Autodesk Inventor part; units mm, degrees
ref_plane "YZ Plane" through (0, 0, 0) normal (1, 0, 0) x (0, 1, 0)
ref_plane "XZ Plane" through (0, 0, 0) normal (0, 1, 0) x (-1, 0, 0)
ref_plane "XY Plane" through (0, 0, 0) normal (0, 0, 1) x (1, 0, 0)
sketch "Sketch1" plane through (0, 0, 0) normal (0, 0, 1) x (1, 0, 0)
  line L0 (-9, 25) -> (9, 25)
  line L1 (9, 25) -> (9, -25)
  line L2 (9, -25) -> (-9, -25)
  line L3 (-9, -25) -> (-9, 25)
  point P0 (0, 0)
  point P1 (0, 25)
  point P2 (-9, 0)
  dimension "d0" = 18
  dimension "d1" = 50
extrude "Extrusion1" add sketch "Sketch1" along normal blind 3
fillet "Fillet1" radius 5 2 edges at (-9, -25, 1.5) (9, -25, 1.5)
fillet "Fillet2" radius 5 2 edges at (-9, 25, 1.5) (9, 25, 1.5)
sketch "Sketch2" plane through (0, 0, 3) normal (0, 0, 1) x (1, 0, 0)
  circle A0 centre (0, -16) radius 9
  circle A1 centre (0, 16) radius 9
  line L0 (-4, -25) -> (4, -25)
  circle A2 centre (0, -8.304) radius 0.75
  line L1 (4, 25) -> (-4, 25)
  point P0 (0, 0)
  dimension "d6" = 18
  dimension "d8" = 1.5
  dimension "d10" = 18
extrude "Extrusion2" cut sketch "Sketch2" against normal up to surface (3 mm away) contours A2
pattern_circular "Circular Pattern1" count 12 over 360 about axis through (0, -16, 3) along (0, 0, 1) of "Extrusion2"
sketch "Sketch4" plane through (0, 0, 3) normal (0, 0, 1) x (1, 0, 0)
  line L0 (-11, 5) -> (9, 5)
  line L1 (9, 5) -> (9, 50)
  line L2 (9, 50) -> (-11, 50)
  line L3 (-11, 50) -> (-11, 5)
  line L4 (-9, 20) -> (-9, -20)
  line L5 (4, 25) -> (-4, 25)
  line L6 (9, -20) -> (9, 20)
  point P0 (0, 0)
  dimension "d25" = 20
  dimension "d26" = 45
  dimension "d27" = 20
extrude "Extrusion5" add sketch "Sketch4" along normal blind 6
sketch "Sketch5" plane through (0, 0, 3) normal (0, 0, 1) x (1, 0, 0)
  line L0 (9, 50) -> (-11, 50)
  line L1 (-5, 5) -> (-11, 5)
  line L2 (-11, 5) -> (-11, 50)
  line L3 (-11, 50) -> (-5, 50)
  line L4 (-5, 50) -> (-5, 5)
  line L5 (-11, 50) -> (-11, 5)
  point P0 (0, 0)
  dimension "d30" = 6
extrude "Extrusion6" add sketch "Sketch5" along normal blind 28
sketch "Sketch6" plane through (-11, 5, 3) normal (-1, 0, 0) x (0, 0, 1)
  circle A0 centre (25, 4) radius 1
  circle A1 centre (9, 4) radius 1
  circle A2 centre (25, 41) radius 1
  circle A3 centre (9, 41) radius 1
  line L0 (0, 0) -> (28, 0)
  line L1 (25, 4) -> (25, 41) construction
  line L2 (28, 45) -> (28, 0)
  point P0 (-3, -5)
  point P1 (28, 22.5)
  point P2 (25, 22.5)
  point P3 (6, 0)
  dimension "d33" = 2
  dimension "d34" = 2
  dimension "d35" = 2
  dimension "d36" = 2
  dimension "d37" = 37
  dimension "d38" = 16
  dimension "d40" = 16
  dimension "d43" = 3
extrude "Extrusion7" cut sketch "Sketch6" against normal up to surface (20 mm away)
properties part number "first_man_link"
Geometry: final body of the model. Coordinates: model frame, mm. A direction names the side the tool comes from. Round coordinates to 2 decimals unless told otherwise and drop trailing zeros. Order: outer loops, then holes, each group sorted by start corner. A loop starts at its lowest first (then second) coordinate and runs counter-clockwise, first axis right, second up. Notation, with made-up numbers: (22, -0.75) -> (37, -0.75) arc R25 ccw to (37, 26.25) -> close; hole circle Ø3 at (56, 57). An arc over 180 degrees is marked (long way). Use one line per item in the form item = value.
(1) Section B-B on z = 12. Return loops of the section in (x, y).
Results list:
outline = (-11, 5) -> (-5, 5) -> (-5, 8) -> (-11, 8) -> close; (-11, 10) -> (-5, 10) -> (-5, 45) -> (-11, 45) -> close; (-11, 47) -> (-5, 47) -> (-5, 50) -> (-11, 50) -> close
(2) Access query for faces 5 (the face through (0, -10, 3)), 6 (the face through (-5, 28, 20)), 7 (the face through (-9, 0, 1)). Directions: +Z, -Z, +X, -X, +Y, -Y. A direction counts if a zero-diameter tool reaches every point of the face in a straight line with its end or side. Return the directions, or none.
Results list:
face_5 = +Z, +X, -X, -Y
face_6 = +Z, +X, +Y, -Y
face_7 = -Z, -X, +Y, -Y
(3) Section C-C on x = 0. Return loops of the section in (y, z), and give its area (3 significant figures).
Results list:
outline = (-25, 0) -> (-24.45, 0) -> (-24.45, 3) -> (-25, 3) -> close; (-22.95, 0) -> (-9.05, 0) -> (-9.05, 3) -> (-22.95, 3) -> close; (-7.55, 0) -> (25, 0) -> (25, 3) -> (50, 3) -> (50, 9) -> (5, 9) -> (5, 3) -> (-7.55, 3) -> close
area = 411 mm^2
(4) Draft query along Y for faces 1 (the face through (9, 15, 4)), 2 (the face through (6.763, -12.896, 1.521)), 3 (the face through (7, -24, 2)), 4 (the face through (-6.07, -11.696, 1.521)). Return one class per face: pulls with the +Y half, pulls with the -Y half, needs draft (parallel to the pull), parting line crosses it, or undercut.
Results list:
face_1 = needs draft
face_2 = undercut
face_3 = pulls with the -Y half
face_4 = undercut
(5) Section A-A on y = 46. Return loops of the section in (x, z).
Results list:
outline = (-11, 3) -> (9, 3) -> (9, 9) -> (-5, 9) -> (-5, 11) -> (-11, 11) -> close; (-11, 13) -> (-5, 13) -> (-5, 27) -> (-11, 27) -> close; (-11, 29) -> (-5, 29) -> (-5, 31) -> (-11, 31) -> close
(6) Ray query, probe 1 along Y at (x, z) = (0, 0.75); probe 2 along Y at (x, z) = (-8.3, 12); probe 3 along Y at (x, z) = (-5.25, 10). Return the intervals inside material, ascending. Write a range as [from, to].
Results list:
probe_1 = [-25, -24.45], [-22.95, -9.05], [-7.55, 25]
probe_2 = [5, 8], [10, 45], [47, 50]
probe_3 = [5, 50]
(7) Section D-D on y = 16.5. Return loops of the section in (x, z), and give its area (3 significant figures).
Results list:
outline = (-11, 3) -> (-9, 3) -> (-9, 0) -> (9, 0) -> (9, 9) -> (-5, 9) -> (-5, 31) -> (-11, 31) -> close
area = 306 mm^2
(8) First-contact query: pin 1 Ø1 at (y, z) = (22, 25) entering from +X; pin 2 Ø8 at (x, z) = (-8.5, 16.5) entering from -Y; pin 3 Ø1.2 at (x, y) = (0, -8.304) entering from +Z; pin 4 Ø2 at (x, y) = (4, -7.5) entering from +Z. Flat tips, straight axial feed; report the tip coordinate or a pass-through.
Results list:
pin_1 = -5
pin_2 = 5
pin_3 = through
pin_4 = 3
